Build history of the part. All positions in model axes, mm. Face numbers are marked on the shaded views. Round coordinates to 2 decimals unless told otherwise and drop trailing zeros. Write each loop counter-clockwise with the first axis right and the second up, starting at its lowest first coordinate (ties: lowest second). Pieces come first, ordered by that corner, then holes.
1) Saw through at C-C (z = 0.85). Write the cut outline in (x, y).
2) Pull direction X, two halves, no side cores. Call the marked faces 1, 2 and 3: +X half, -X half, draft (parallel to the pull), parting line (faces both ways), or undercut.
3) Saw through at A-A (x = 0). Write the cut outline in (y, z), plus the area to 3 significant figures.
4) Saw through at B-B (y = 0). Write the cut outline in (x, z).
5) Wall check: probe 1 along Y at (x, z) = (0, 0.9); probe 2 along X at (y, z) = (0.75, 1.95). Give the ranges that are in metal, low to high.
6) Saw through at D-D (x = 4). Write the cut outline in (y, z).
7) Flat gauge pin, fed straight in: pin 1 (3 mm diameter, centred on x = -2, y = -1, fed in from -Z). Where does the tip first touch, or does it go through?
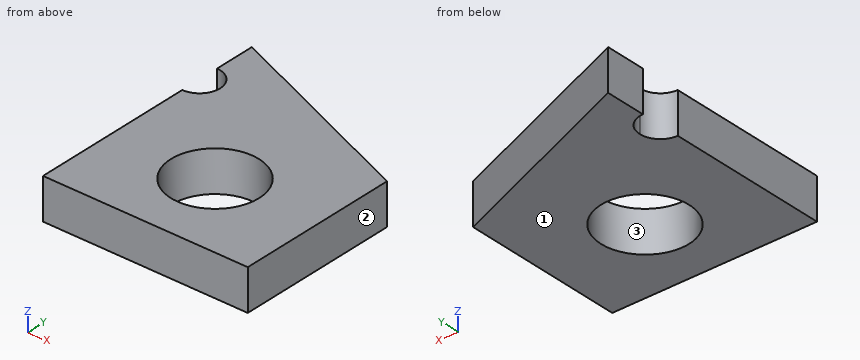
from build123d import *

# Parameters (mm, degrees)
F0_W     = 12.7
F0_H     = 10.16
F1_DEPTH = 2.54
F3_DEPTH = 25.4
F4_R     = 2.7305
F5_DEPTH = 25.4


with BuildPart() as f1:
    # F0 (on Top) → F1 (new body)
    with BuildSketch(Plane.XY):
        Rectangle(F0_W, F0_H)
        Polygon((-6.35, 5.08), (6.35, 5.08), (-6.35, 10.16), align=None)
    extrude(amount=F1_DEPTH)

    # F2 (on face) → F3 (cut)
    with BuildSketch(Plane.XY.offset(2.54)):
        with BuildLine():
            ThreePointArc((-6.35, 5.08), (-5.451974, 5.451974), (-5.08, 6.35))
            ThreePointArc((-5.08, 6.35), (-7.248026, 7.248026), (-6.35, 5.08))
        make_face()
    extrude(amount=-F3_DEPTH, mode=Mode.SUBTRACT)

    # F4 (on face) → F5 (cut)
    with BuildSketch(Plane.XY.offset(2.54)):
        Circle(F4_R)
    extrude(amount=-F5_DEPTH, mode=Mode.SUBTRACT)


solid = f1.part
Evaluation:
1. outline: (-6.35, -5.08) - (6.35, -5.08) - (6.35, 5.08) - (-6.35, 10.16) - (-6.35, 7.62) arc R1.27 cw to (-5.08, 6.35) arc R1.27 cw to (-6.35, 5.08) - close; hole circle Ø5.46 at (0, 0)
2. face 1: draft
2. face 2: +X half
2. face 3: undercut
3. outline: (-5.08, 0) - (-2.73, 0) - (-2.73, 2.54) - (-5.08, 2.54) - close; (2.73, 0) - (7.62, 0) - (7.62, 2.54) - (2.73, 2.54) - close
3. area: 18.4 mm2
4. outline: (-6.35, 0) - (-2.73, 0) - (-2.73, 2.54) - (-6.35, 2.54) - close; (2.73, 0) - (6.35, 0) - (6.35, 2.54) - (2.73, 2.54) - close
5. probe 1: y = -5.08 to -2.73, 2.73 to 7.62
5. probe 2: x = -6.35 to -2.63, 2.63 to 6.35
6. outline: (-5.08, 0) - (6.02, 0) - (6.02, 2.54) - (-5.08, 2.54) - close
7. pin 1: stops at z = 0
